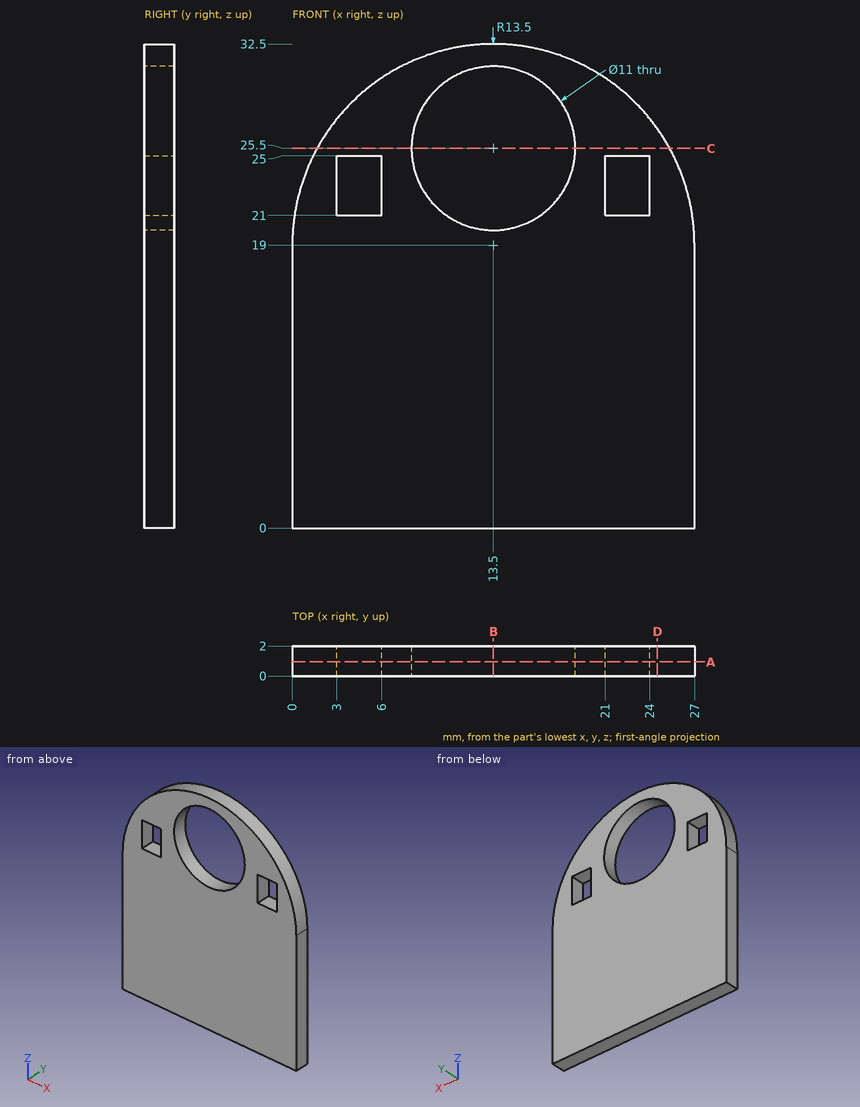
Job drawing, mm, ordinate dimensions from the low corner. One solid piece. Round coordinates to 2 decimals unless told otherwise and drop trailing zeros. Write each loop counter-clockwise with the first axis right and the second up, starting at its lowest first coordinate (ties: lowest second). Pieces come first, ordered by that corner, then holes.
1) Drill centre lines: probe 1 along Z at (x, y) = (13.5, 1.25); probe 2 along X at (y, z) = (0.2, 23); probe 3 along Z at (x, y) = (18, 0.35). Where is each one in solid material? Low to high.
2) Band-saw the part on C-C, the plane z = 25.5. List the corners of the cut face in (x, y).
3) Band-saw the part on A-A, the plane y = 0.95. List the corners of the cut face in (x, z).
4) Band-saw the part on B-B, the plane x = 13.5. List the corners of the cut face in (y, z), and give its area (3 significant figures).
5) Band-saw the part on D-D, the plane x = 24.5. List the corners of the cut face in (y, z), and give its area (3 significant figures).
6) Pin check, flat tips, straight feed: pin 1 (0.6 mm diameter, centred on y = 1, z = 23, fed in from +X); pin 2 (1 mm diameter, centred on y = 1, z = 24, fed in from -X); pin 3 (0.6 mm diameter, centred on y = 1, z = 23.5, fed in from +X); pin 4 (9 mm diameter, centred on x = 13.5, z = 25.5, fed in from +Y). Stop position of each tip, or through.
Ans:
1. probe 1: z = 0 to 20, 31 to 32.5
1. probe 2: x = 0.61 to 3, 6 to 8.6, 18.4 to 21, 24 to 26.39
1. probe 3: z = 0 to 22.34, 28.66 to 31.73
2. outline: (1.67, 0) - (8, 0) - (8, 2) - (1.67, 2) - close; (19, 0) - (25.33, 0) - (25.33, 2) - (19, 2) - close
3. outline: (0, 0) - (27, 0) - (27, 19) arc R13.5 ccw to (0, 19) - close; hole (3, 21) - (6, 21) - (6, 25) - (3, 25) - close; hole circle Ø11 at (13.5, 25.5); hole (21, 21) - (24, 21) - (24, 25) - (21, 25) - close
4. outline: (0, 0) - (2, 0) - (2, 20) - (0, 20) - close; (0, 31) - (2, 31) - (2, 32.5) - (0, 32.5) - close
4. area: 43.0 mm2
5. outline: (0, 0) - (2, 0) - (2, 26.83) - (0, 26.83) - close
5. area: 53.7 mm2
6. pin 1: stops at x = 26.48
6. pin 2: stops at x = 0.77
6. pin 3: stops at x = 26.33
6. pin 4: passes through
